from build123d import *

# Parameters (mm, degrees)
SKETCH1_R             = 6
BOSS_EXTRUDE1_DEPTH   = 10
BOSS_EXTRUDE1_2_DEPTH = 10
SKETCH1_3_R           = 6
SKETCH1_3_R_2         = 15
BOSS_EXTRUDE2_DEPTH   = 5


with BuildPart() as part:
    # Sketch1 → Boss-Extrude1 (new, symmetric)
    with BuildSketch(Plane.XY):
        with BuildLine():
            Line((-55.432771951, 22.961005942), (-69.290964938, 28.701257427))
            ThreePointArc((-69.290964938, 28.701257427), (-53.033008589, 53.033008589), (-28.701257427, 69.290964938))
            Line((-28.701257427, 69.290964938), (-9.567085809, 23.096988313))
            ThreePointArc((-9.567085809, 23.096988313), (-17.510562404, 17.843211715), (-22.912878475, 10))
            Line((-22.912878475, 10), (-17.320508076, 10))
            ThreePointArc((-17.320508076, 10), (-20, 0), (-17.320508076, -10))
            Line((-17.320508076, -10), (-22.912878475, -10))
            ThreePointArc((-22.912878475, -10), (-17.510562404, -17.843211715), (-9.567085809, -23.096988313))
            Line((-9.567085809, -23.096988313), (-28.701257427, -69.290964938))
            ThreePointArc((-28.701257427, -69.290964938), (-53.033008589, -53.033008589), (-69.290964938, -28.701257427))
            Line((-69.290964938, -28.701257427), (-55.432771951, -22.961005942))
            ThreePointArc((-55.432771951, -22.961005942), (-60, 0), (-55.432771951, 22.961005942))
        make_face()
        with Locations((-28.284271247, -28.284271247)):
            Circle(SKETCH1_R, mode=Mode.SUBTRACT)
        with Locations((-40, 0)):
            Circle(SKETCH1_R, mode=Mode.SUBTRACT)
        with Locations((-28.284271247, 28.284271247)):
            Circle(SKETCH1_R, mode=Mode.SUBTRACT)
    extrude(amount=BOSS_EXTRUDE1_DEPTH, both=True)



with BuildPart() as body_2:
    # Sketch1 → Boss-Extrude1 2 (new, symmetric)
    with BuildSketch(Plane.XY):
        with BuildLine():
            Line((55.432771951, -22.961005942), (69.290964938, -28.701257427))
            ThreePointArc((69.290964938, -28.701257427), (53.033008589, -53.033008589), (28.701257427, -69.290964938))
            Line((28.701257427, -69.290964938), (9.567085809, -23.096988313))
            ThreePointArc((9.567085809, -23.096988313), (17.510562404, -17.843211715), (22.912878475, -10))
            Line((22.912878475, -10), (17.320508076, -10))
            ThreePointArc((17.320508076, -10), (20, 0), (17.320508076, 10))
            Line((17.320508076, 10), (22.912878475, 10))
            ThreePointArc((22.912878475, 10), (17.510562404, 17.843211715), (9.567085809, 23.096988313))
            Line((9.567085809, 23.096988313), (28.701257427, 69.290964938))
            ThreePointArc((28.701257427, 69.290964938), (53.033008589, 53.033008589), (69.290964938, 28.701257427))
            Line((69.290964938, 28.701257427), (55.432771951, 22.961005942))
            ThreePointArc((55.432771951, 22.961005942), (60, 0), (55.432771951, -22.961005942))
        make_face()
        with Locations((28.284271247, 28.284271247)):
            Circle(SKETCH1_R, mode=Mode.SUBTRACT)
        with Locations((40, 0)):
            Circle(SKETCH1_R, mode=Mode.SUBTRACT)
        with Locations((28.284271247, -28.284271247)):
            Circle(SKETCH1_R, mode=Mode.SUBTRACT)
    extrude(amount=BOSS_EXTRUDE1_2_DEPTH, both=True)


with BuildPart() as part_1:
    add(part.part)

    add(body_2.part)  # Boss-Extrude2 merges body 2
    # Sketch1_3 → Boss-Extrude2 (add, symmetric)
    with BuildSketch(Plane.XY):
        with BuildLine():
            ThreePointArc((22.912878475, 10), (17.510562404, 17.843211715), (9.567085809, 23.096988313))
            Line((9.567085809, 23.096988313), (22.961005942, 55.432771951))
            ThreePointArc((22.961005942, 55.432771951), (0, 60), (-22.961005942, 55.432771951))
            Line((-22.961005942, 55.432771951), (-9.567085809, 23.096988313))
            ThreePointArc((-9.567085809, 23.096988313), (-17.510562404, 17.843211715), (-22.912878475, 10))
            Line((-22.912878475, 10), (-17.320508076, 10))
            ThreePointArc((-17.320508076, 10), (-20, 0), (-17.320508076, -10))
            Line((-17.320508076, -10), (-22.912878475, -10))
            ThreePointArc((-22.912878475, -10), (-17.510562404, -17.843211715), (-9.567085809, -23.096988313))
            Line((-9.567085809, -23.096988313), (-22.961005942, -55.432771951))
            ThreePointArc((-22.961005942, -55.432771951), (0, -60), (22.961005942, -55.432771951))
            Line((22.961005942, -55.432771951), (9.567085809, -23.096988313))
            ThreePointArc((9.567085809, -23.096988313), (17.510562404, -17.843211715), (22.912878475, -10))
            Line((22.912878475, -10), (17.320508076, -10))
            ThreePointArc((17.320508076, -10), (20, 0), (17.320508076, 10))
            Line((17.320508076, 10), (22.912878475, 10))
        make_face()
        with Locations((0, -40)):
            Circle(SKETCH1_3_R, mode=Mode.SUBTRACT)
        Circle(SKETCH1_3_R_2, mode=Mode.SUBTRACT)
        with Locations((0, 40)):
            Circle(SKETCH1_3_R, mode=Mode.SUBTRACT)
    extrude(amount=BOSS_EXTRUDE2_DEPTH, both=True)


solid = part_1.part
The listing builds one solid part. Answer for the finished solid, in the listing's coordinates (mm). A direction names the side the tool comes from. Give positions to 0.01 mm unless a question says otherwise; leave off trailing zeros. Loops run counter-clockwise (first coordinate to the right, second up) from the corner with the lowest first, then second, coordinate; pieces in that order, holes last.
Item 1: A tool of negligible diameter and unlimited length cuts with its end or side. For faces 4 (the cylindrical face through (-20, 0, 8)), 5 (the flat face through (-62.46, -25.87, 0.14)), 6 (the cylindrical face through (-22.74, 25.99, -0.14)), 7 (the flat face through (62.46, 25.87, 0.14)), 8 (the flat face through (-20, -10, -7)), from which of +Z, -Z, +X, -X, +Y, -Y can it reach the whole face along a straight path? Write none if from no direction.
Derived:
face 4: +Z
face 5: +Z, -Z, -X
face 6: +Z, -Z
face 7: +Z, -Z, +X
face 8: -Z
Item 2: Each of these flat-tipped pins is pushed along its axis until it touches: pin 1 Ø5.5 at (x, z) = (19.5, 7) entering from -Y; pin 2 Ø10 at (x, z) = (15, 2) entering from +Y; pin 3 Ø10 at (y, z) = (-7.5, 3) entering from -X; pin 4 Ø7 at (x, y) = (28.28, 28.28) entering from -Z. Where does it stop, or does it pass through?
Derived:
pin 1: stops at y = -57.36
pin 2: stops at y = 59.16
pin 3: stops at x = -59.95
pin 4: passes through
Item 3: Determine the mould class of faces 1 (the flat face through (20, -10, 8)), 2 (the flat face through (-23.52, 56.78, 0.14)), 3 (the cylindrical face through (-52.741, -53.324, 0.14)) for opening direction Y: +Y half, -Y half, draft (parallel to the pull), parting line (faces both ways), or undercut.
Derived:
face 1: undercut
face 2: +Y half
face 3: -Y half
Item 4: A cutting plane is placed at B-B (x = 0). Give the vertices of the cut face in (y, z).
Derived:
outline: (-60, -5) - (-46, -5) - (-46, 5) - (-60, 5) - close; (-34, -5) - (-15, -5) - (-15, 5) - (-34, 5) - close; (15, -5) - (34, -5) - (34, 5) - (15, 5) - close; (46, -5) - (60, -5) - (60, 5) - (46, 5) - close
Item 5: Find the intervals of material crossed by line 1 along Y through (x, z) = (0, 0.75); line 2 along Y through (x, z) = (-28.5, -1); line 3 along Y through (x, z) = (-26, -1.75), in increasing order.
Derived:
line 1: y = -60 to -46, -34 to -15, 15 to 34, 46 to 60
line 2: y = -68.81 to -34.28, -22.29 to 22.29, 34.28 to 68.81
line 3: y = -62.77 to -33.83, -22.74 to 22.74, 33.83 to 62.77
Item 6: A cutting plane is placed at A-A (y = 0). Give the vertices of the cut face in (x, z), then the cut area to 3 significant figures.
Derived:
outline: (-60, -10) - (-46, -10) - (-46, 10) - (-60, 10) - close; (-34, -10) - (-20, -10) - (-20, -5) - (-15, -5) - (-15, 5) - (-20, 5) - (-20, 10) - (-34, 10) - close; (15, -5) - (20, -5) - (20, -10) - (34, -10) - (34, 10) - (20, 10) - (20, 5) - (15, 5) - close; (46, -10) - (60, -10) - (60, 10) - (46, 10) - close
area: 1,220 mm2
Item 7: A cutting plane is placed at C-C (z = -3). Give the number of separate pieces and of enclosed holes in the cut face, then the cut area to 3 significant figures.
Derived:
separate pieces: 1
enclosed holes: 9
area: 12,900 mm2
